```python
from build123d import *

# Parameters (mm, degrees)
F0_W     = 50
F0_H     = 50
F5_W     = 45.6
F5_H     = 45.6
F6_DEPTH = 3


with BuildPart() as f2:
    # F0 (on Top) → F2 section 0
    with BuildSketch(Plane.XY, mode=Mode.PRIVATE) as f2_s0:
        Rectangle(F0_W, F0_H)
    loft([f2_s0.sketch, Vertex(0, 0, 45.518458)])

    # F3 (on Right) → F4 (revolve)
    with BuildSketch(Plane.YZ):
        with BuildLine():
            Line((0, 41.007266), (0, 56.007266))
            ThreePointArc((0, 56.007266), (-7.5, 48.507266), (0, 41.007266))
        make_face()
    revolve(axis=Axis((0, 0, 48.507266), (0, 0, -1)))

    # F5 (on Top) → F6 (join)
    with BuildSketch(Plane.XY):
        Rectangle(F5_W, F5_H)
    extrude(amount=-F6_DEPTH)


solid = f2.part
```
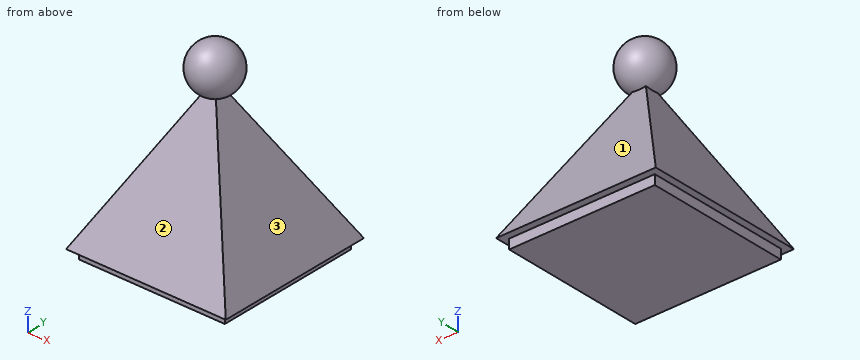
Here's how the part is built. I have some questions about the finished solid (model axes, mm). Face numbers are marked on the shaded views. Coordinates: 2 decimals unless noted, no trailing zeros. Loops run counter-clockwise (first coordinate to the right, second up) from the corner with the lowest first, then second, coordinate; pieces in that order, holes last. Notation, with made-up numbers: (77, -40) -> (102, -40) arc R26 ccw to (102, -20) -> close; hole circle Ø8 at (66.5, -13). An arc over 180 degrees is marked (long way). Return JSON: item names as keys, results as strings.
1) Thinking about a two-plate mould opening in Y: for the marked faces 1, 2 and 3, which applies, +Y half, -Y half, draft (parallel to the pull), parting line (faces both ways), or undercut?
Results below:
{"face 1": "+Y half", "face 2": "-Y half", "face 3": "draft"}
2) I need wall thicknesses on line 1 (Z direction, x = 1, y = 5.5); line 2 (Y direction, x = 9.5, z = -0.5); line 3 (Y direction, x = -3, z = 48.5). Which ranges of each line are inside material? Lowest first, please. Write a range as from..to.
Results below:
{"line 1": "-3..35.5, 43.51..53.51", "line 2": "-22.8..22.8", "line 3": "-6.87..6.87"}
3) If we section it at C-C, the plane x = -11: Write out the boundary of the cut face in (y, z).
Results below:
{"outline": "(-25, 0) -> (-22.8, 0) -> (-22.8, -3) -> (22.8, -3) -> (22.8, 0) -> (25, 0) -> (11, 25.49) -> (-11, 25.49) -> close"}
4) If we section it at D-D, the plane y = -10: Write out the boundary of the cut face in (x, z), then the cut area to 3 significant figures.
Results below:
{"outline": "(-25, 0) -> (-22.8, 0) -> (-22.8, -3) -> (22.8, -3) -> (22.8, 0) -> (25, 0) -> (10, 27.31) -> (-10, 27.31) -> close", "area": "1,090 mm²"}
5) If we section it at B-B, the plane y = 5: Write out the boundary of the cut face in (x, z), then the cut area to 3 significant figures.
Results below:
{"outline": "(-25, 0) -> (-22.8, 0) -> (-22.8, -3) -> (22.8, -3) -> (22.8, 0) -> (25, 0) -> (5, 36.41) -> (-5, 36.41) -> close; circle Ø11.18 at (0, 48.51)", "area": "1,330 mm²"}
6) Will these pins go through, and if not, where does the flat tip stop? pin 1 (2 mm diameter, centred on x = -11.5, z = 18.5, fed in from -Y); pin 2 (2.5 mm diameter, centred on y = -8, z = -1, fed in from -X); pin 3 (4 mm diameter, centred on y = -15.5, z = 8.5, fed in from +X); pin 4 (8 mm diameter, centred on y = -3, z = 24, fed in from +X).
Results below:
{"pin 1": "y = -15.39", "pin 2": "x = -25", "pin 3": "x = 21.43", "pin 4": "x = 14.02"}
7) If we section it at A-A, the plane x = -3: Write out the boundary of the cut face in (y, z).
Results below:
{"outline": "(-25, 0) -> (-22.8, 0) -> (-22.8, -3) -> (22.8, -3) -> (22.8, 0) -> (25, 0) -> (3, 40.06) -> (-3, 40.06) -> close; circle Ø13.75 at (0, 48.51)"}
